Autodesk Fusion 360 part; units mm, degrees
sketch "Sketch1" plane through (0, 0, 0) normal (0, 0, 1) x (1, 0, 0)
  line L0 (0, 0) -> (20, 0)
  line L1 (20, 0) -> (20, 25)
  line L2 (20, 25) -> (0, 25)
  line L3 (0, 25) -> (0, 0)
extrude "Extrude1" add sketch "Sketch1" along normal blind 20
sketch "Sketch2" plane through (0, 0, 0) normal (0, 0, -1) x (1, 0, 0)
  line L0 (0, 0) -> (0, -25)
  line L1 (0, -25) -> (20, -25)
  line L2 (20, -25) -> (20, 0)
  line L3 (20, 0) -> (0, 0)
shell "Shell1" thickness 2 removed faces 0 bodies 1
sketch "Sketch3" plane through (0, 0, 20) normal (0, 0, 1) x (-1, 0, 0)
  line L0 (0, -25) -> (0, 0)
  line L1 (0, 0) -> (-20, 0)
  line L2 (-20, 0) -> (-20, -25)
  line L3 (-20, -25) -> (0, -25)
hole "Hole1" at (9.9202, 12.4035, 20) direction (0, 0, -1) diameter 3 depth 25 tip angle 118
hole "Hole2" at (9.8027, 0, 10.2267) direction (0, 1, 0) diameter 9 depth 4 tip angle 118
sketch "Sketch4" plane through (20, 0, 0) normal (1, 0, 0) x (0, 1, 0)
  line L0 (0, 0) -> (25, 0)
  line L1 (25, 0) -> (25, 20)
  line L2 (25, 20) -> (0, 20)
  line L3 (0, 20) -> (0, 0)
  line L4 (12.5, 0.7539) -> (2, 2)
  line L5 (2, 2) -> (23, 2)
  line L6 (23, 2) -> (12.5, 0.7539)
  line L7 (2, 2) -> (23, 2)
  line L8 (2, 2) -> (12.5, 0.7539)
  line L9 (23, 2) -> (12.5, 0.7539)
extrude "Extrude2" cut sketch "Sketch4" against normal blind 18 from surface at -1 contours L4 L5 L6 L7 L8 L9
ref_plane "WorkPlane1" through (0, 0, 20) normal (0.6155, -0.4924, 0.6155) x (0.6247, 0.7809, 0)
ref_plane "WorkPlane2" through (15, 12.5, 10) normal (1, 0, 0) x (0, 1, 0)
sketch "Sketch7" plane through (15, 0, 0) normal (1, 0, 0) x (0, 1, 0)
  line L0 (-2, 22) -> (31, 22)
  line L1 (31, 22) -> (31, -5)
  line L2 (31, -5) -> (-2, -5)
  line L3 (-2, -5) -> (-2, 22)
sketch "Sketch6" plane through (7.5758, -6.0606, 7.5758) normal (0.6155, -0.4924, 0.6155) x (0.6247, 0.7809, 0)
  line L0 (-4, 34) -> (46, 34)
  line L1 (46, 34) -> (46, -16)
  line L2 (46, -16) -> (-4, -16)
  line L3 (-4, -16) -> (-4, 34)
extrude "Extrude3" [suppressed]
sketch "Sketch5" plane through (0, 25, 0) normal (0, 1, 0) x (-1, 0, 0)
  line L0 (-20, 0) -> (0, 0)
  line L1 (0, 0) -> (0, 20)
  line L2 (0, 20) -> (-20, 20)
  line L3 (-20, 20) -> (-20, 0)
  line L4 (-10, 0.754) -> (-18, 2)
  line L5 (-18, 2) -> (-2, 2)
  line L6 (-2, 2) -> (-10, 0.754)
Design review of the part built by this model. Coordinates are the model's own, in mm. A direction names the side the tool comes from. Coordinates: 2 decimals unless noted, no trailing zeros. Order: outer loops, then holes, each group sorted by start corner. A loop starts at its lowest first (then second) coordinate and runs counter-clockwise, first axis right, second up. Notation, with made-up numbers: (51.25, -21) -> (56.25, -21) arc R17 ccw to (56.25, 0) -> close; hole circle Ø11 at (60, 75.25). An arc over 180 degrees is marked (long way). Use one line per item in the form item = value. Start each with the question number.
(1) The part is to be moulded in two halves that separate along Z. For faces 1 (the flat face through (20, 12, 10)), 2 (the flat face through (12, 13, 20)), 3 (the flat face through (18.5, 12.4, 2)), say which applies: +Z half, -Z half, draft (parallel to the pull), parting line (faces both ways), or undercut.
(2) Add section A-A on z = 16.5. State the section outline as (x, y) points.
(3) Add section D-D on x = 11. State the section outline as (y, z) points, plus the area to 3 significant figures.
(4) Insertion check: pin 1 (2.5 mm diameter, centred on x = 9.92, y = 12.4, fed in from +Z). The pin has a flat end and moves straight along its axis. Give the tip position at first contact, or say it passes through.
(5) For probe 1 along Y at (x, z) = (4, 13.75); probe 2 along X at (y, z) = (7.75, 6.5); probe 3 along X at (y, z) = (11, 1.75), list the stretches that pass through material, from the lowest coordinate up.
(6) Add section C-C on y = 15. State the section outline as (x, z) points.
(7) Add section B-B on x = 4.5. State the section outline as (y, z) points.
(8) For faces 4 (the cylindrical face through (5.34, 1.01, 10.81)), 5 (the cylindrical face through (11.25, 11.71, 0.47)), 6 (the flat face through (19, 12.4, 1.5)), list the 3-axis set-ups (+Z, -Z, +X, -X, +Y, -Y) from which the entire face can be reached by the end or side of a thin tool; tool diameter is ignored.
Answer block:
q1.face_1 = draft
q1.face_2 = +Z half
q1.face_3 = undercut
q2.outline = (0, 0) -> (20, 0) -> (20, 25) -> (0, 25) -> close; hole (2, 2) -> (18, 2) -> (18, 23) -> (2, 23) -> close
q3.outline = (0, 0) -> (11.36, 0) -> (11.36, 0.89) -> (2, 2) -> (2, 5.89) -> (0, 5.89) -> close; (0, 14.56) -> (2, 14.56) -> (2, 18) -> (11.36, 18) -> (11.36, 20) -> (0, 20) -> close; (13.44, 0) -> (25, 0) -> (25, 20) -> (13.44, 20) -> (13.44, 18) -> (23, 18) -> (23, 2) -> (13.44, 0.87) -> close
q3.area = 128 mm²
q4.pin_1 = through
q5.probe_1 = 0 to 2, 23 to 25
q5.probe_2 = 0 to 2, 18 to 20
q5.probe_3 = 0 to 1, 19 to 20
q6.outline = (0, 0) -> (20, 0) -> (20, 20) -> (0, 20) -> close; hole (1, 1.05) -> (19, 1.05) -> (19, 2) -> (18, 2) -> (18, 18) -> (2, 18) -> (2, 2) -> (1, 2) -> close
q7.outline = (0, 0) -> (25, 0) -> (25, 20) -> (0, 20) -> close; hole (2, 2) -> (12.5, 0.75) -> (23, 2) -> (23, 18) -> (2, 18) -> close
q8.face_4 = -Y
q8.face_5 = +Z, -Z
q8.face_6 = none
